Work out the finished part from the listing and answer in its coordinate system (mm). A direction names the side the tool comes from. Give positions to 0.01 mm unless a question says otherwise; leave off trailing zeros. Loops run counter-clockwise (first coordinate to the right, second up) from the corner with the lowest first, then second, coordinate; pieces in that order, holes last. Notation, with made-up numbers: M 8.5,47.25 L 25.5,47.25 A33 cw 25.5,80.25 Z; hole C 41,-1.75 d5. An arc over 180 degrees is marked long. Answer in a Markdown table with one row per item. Add a question column.
from build123d import *

# Parameters (mm, degrees)
SKETCH_1_R      = 8
EXTRUDE_1_DEPTH = 5
FILLET_1_R      = 0.5


with BuildPart() as part:
    # 草图1 → 凸台-拉伸1 (new body)
    with BuildSketch(Plane.XY):
        with BuildLine():
            Line((-8, 19.305502441), (-8, 100.694497559))
            ThreePointArc((-8, 100.694497559), (-8.829546885, 104.682327755), (-11.180557935, 108.008539527))
            ThreePointArc((-11.180557935, 108.008539527), (0.051988176, 136.395038799), (11.104284737, 107.93787496))
            ThreePointArc((11.104284737, 107.93787496), (8.732226543, 104.626639898), (7.877406014, 100.644150781))
            Line((7.877406014, 100.644150781), (7.365590706, 19.941690023))
            ThreePointArc((7.365590706, 19.941690023), (8.247647691, 15.771352421), (10.786374698, 12.347231304))
            ThreePointArc((10.786374698, 12.347231304), (0.265496379, -16.392971411), (-11.180557935, 11.991460473))
            ThreePointArc((-11.180557935, 11.991460473), (-8.829546885, 15.317672245), (-8, 19.305502441))
        make_face()
        with Locations((0, 120)):
            Circle(SKETCH_1_R, mode=Mode.SUBTRACT)
        Circle(SKETCH_1_R, mode=Mode.SUBTRACT)
    extrude(amount=EXTRUDE_1_DEPTH)

    # 圆角1
    fillet_1_edges = [part.edges().sort_by_distance(p)[0] for p in [
        (0.265496379, -16.392971411, 0),
        (-8.829546885, 15.317672245, 0),
        (-8, 60, 0),
        (-8.829546885, 104.682327755, 0),
        (-8.829546885, 15.317672245, 5),
        (0.265496379, -16.392971411, 5),
        (8.247647691, 15.771352421, 5),
        (7.62149836, 60.292920402, 5),
        (8.732226543, 104.626639898, 5),
        (0.051988176, 136.395038799, 5),
        (-8.829546885, 104.682327755, 5),
        (0.051988176, 136.395038799, 0),
        (-8, 60, 5),
        (8.732226543, 104.626639898, 0),
        (7.62149836, 60.292920402, 0),
        (8.247647691, 15.771352421, 0),
    ]]
    fillet(fillet_1_edges, radius=FILLET_1_R)


solid = part.part
(1) Each of these flat-tipped pins is pushed along its axis until it touches: P1, Ø2, axis at y = 40.5, z = 3.5, coming from the -X side; P2, Ø1.5, axis at x = 1.5, z = 2.5, coming from the -Y side; P3, Ø1, axis at y = 53.5, z = 3.5, coming from the +X side; P4, Ø9.5, axis at x = 0, y = 120, coming from the -Z side. Where does it stop, or does it pass through?
(2) Section A-A, the plane z = 2.45 is taken. Determine the outline of the cut face in (x, y), and give its area (3 significant figures).
(3) Consider line 1 along Y through (x, z) = (0, 2.65); line 2 along Y through (x, z) = (6, 4.85); line 3 along Y through (x, z) = (9.5, 0.75). Determine where each line is inside the solid, lowest interval first. Write a range as from..to.
(4) The mould has two halves that part along Y. Classify faces 1 (the face through (0, 61, 5)), 2 (the face through (-0.498, 136.388, 2.472)), 3 (the face through (-8, 59, 2)): pulls with the +Y half, pulls with the -Y half, needs draft (parallel to the pull), parting line crosses it, or undercut.
(5) Section B-B, the plane x = 0 is taken. State how many separate pieces and enclosed holes the cut face has, and give its area (3 significant figures).
(6) Which of the six approach directions +Z, -Z, +X, -X, +Y, -Y give full straight-line access (tool end or side, diameter ignored) to faces 4 (the face through (0.818, -16.375, 2.472)), 5 (the face through (-8.85, 15.27, 2.47)), 6 (the face through (8.22, 15.83, 2.47))?
Numbers:
| question | item | result |
|---|---|---|
| 1 | P1 | stops at x = -8 |
| 1 | P2 | stops at y = -16.38 |
| 1 | P3 | stops at x = 7.58 |
| 1 | P4 | passes through |
| 2 | outline | M -11.18,11.99 A16.4 ccw long 10.79,12.35 A10 cw 7.37,19.94 L 7.88,100.64 A10 cw 11.1,107.94 A16.4 ccw long -11.18,108.01 A10 cw -8,100.69 L -8,19.31 A10 cw Z; hole C 0,0 d16; hole C 0,120 d16 |
| 2 | area | 2,680 mm² |
| 3 | line 1 | y = -16.4..-8, 8..112, 128..136.4 |
| 3 | line 2 | y = -15.1..-5.29, 5.29..114.71, 125.29..135.1 |
| 3 | line 3 | y = -13.36..13.7, 106.04..133.36 |
| 4 | face 1 | needs draft |
| 4 | face 2 | undercut |
| 4 | face 3 | undercut |
| 5 | separate pieces | 3 |
| 5 | enclosed holes | 0 |
| 5 | area | 604 mm² |
| 6 | face 4 | +Z, -Z |
| 6 | face 5 | +Z, -Z, -X |
| 6 | face 6 | +Z, -Z, +X |
